```python
from build123d import *

# Parameters (mm, degrees)
SKETCH1_W           = 3
SKETCH1_H           = 400
SKETCH6_OUTSIDE_W   = 208.902
SKETCH6_OUTSIDE_H   = 208.902
CUT_EXTRUDE2_DEPTH  = 409.900966005
BOSS_EXTRUDE4_DEPTH = 7
FILLET1_R           = 10


with BuildPart() as part:
    # Sketch1 → Revolve1 (revolve)
    with BuildSketch(Plane.XY, mode=Mode.PRIVATE) as revolve1_sk:
        with Locations((58.5, 0)):
            Rectangle(SKETCH1_W, SKETCH1_H)
    revolve(revolve1_sk.sketch.rotate(Axis((0, 0, 0), (0, 1, 0)), 90), axis=Axis((0, 0, 0), (0, 1, 0)))

    # Sketch6 outside → Cut-Extrude2 (cut, through all)
    with BuildSketch(Plane(origin=(0, 200, 0), x_dir=(1, 0, 0), z_dir=(0, 1, 0))):
        Rectangle(SKETCH6_OUTSIDE_W, SKETCH6_OUTSIDE_H)
        with BuildLine():
            Line((0, -25.455844123), (53.200134751, 27.744290628))
            ThreePointArc((53.200134751, 27.744290628), (0, 60), (-53.200134751, 27.744290628))
            Line((-53.200134751, 27.744290628), (0, -25.455844123))
        make_face(mode=Mode.SUBTRACT)
    extrude(amount=-CUT_EXTRUDE2_DEPTH, mode=Mode.SUBTRACT)

    # Sketch7 → Boss-Extrude4 (add)
    with BuildSketch(Plane(origin=(0, 200, 0), x_dir=(1, 0, 0), z_dir=(0, 1, 0))):
        with BuildLine():
            Line((-35.629141961, 42.982621722), (-21.797880868, 52.667375003))
            ThreePointArc((-21.797880868, 52.667375003), (-31.660719889, 47.398299717), (-40.305086528, 40.305086528))
            Line((-40.305086528, 40.305086528), (-34.793335026, 34.793335026))
            ThreePointArc((-34.793335026, 34.793335026), (-28.516275136, 41.671387576), (-22.892502884, 49.093130862))
            Line((-22.892502884, 49.093130862), (-34.309916158, 41.09857202))
            ThreePointArc((-34.309916158, 41.09857202), (-35.91155391, 41.380983969), (-35.629141961, 42.982621722))
        make_face()
    boss_extrude4 = extrude(amount=-BOSS_EXTRUDE4_DEPTH)

    # Mirror1: Boss-Extrude4 across plane
    add(boss_extrude4.mirror(Plane.ZX))

    # Fillet1
    fillet1_edges = [part.edges().sort_by_distance(p)[0] for p in [
        (52.085351582, 200, -26.629507459),
        (-52.085351582, -200, -26.629507459),
        (52.085351582, -200, -26.629507459),
        (-52.085351582, 200, -26.629507459),
    ]]
    fillet(fillet1_edges, radius=FILLET1_R)


solid = part.part
```
The model under review builds one solid part; all positions refer to its coordinate system, in mm. A direction names the side the tool comes from. Coordinates: 2 decimals unless noted, no trailing zeros. Order: outer loops, then holes, each group sorted by start corner. A loop starts at its lowest first (then second) coordinate and runs counter-clockwise, first axis right, second up. Notation, with made-up numbers: (2.5, 21) -> (54.5, 21) arc R8 ccw to (54.5, 32) -> close; hole circle Ø9 at (77.25, -18.75). An arc over 180 degrees is marked (long way). Answer in a Markdown table with one row per item. Add a question column.
Item 1: To check wall thickness, follow probe 1 along X at (y, z) = (33, -37); probe 2 along X at (y, z) = (7, -45.5); probe 3 along Z at (x, y) = (44, -108). State the ranges of each line that lie inside material, in increasing order.
Item 2: Mouldability with a two-part tool opening along X and no side actions: class faces 1 (the cylindrical face through (-50.72, 197.15, -29.52)), 2 (the cylindrical face through (50.72, -197.15, -29.52)), 3 (the flat face through (-32, 193, -42)) as +X half, -X half, draft (parallel to the pull), parting line (faces both ways), or undercut.
Item 3: We need section A-A on y = -24.5. Write out the cut boundary in (x, z).
Item 4: We need section B-B on x = 15. Write out the cut boundary in (y, z), plus the area to 3 significant figures.
Item 5: Clearance check with flat-ended pins moving along their axes: pin 1 (1.5 mm diameter, centred on x = 31.5, z = -46.5, fed in from +Y); pin 2 (10 mm diameter, centred on x = 39.5, y = 8.5, fed in from +Z); pin 3 (6 mm diameter, centred on y = 126.5, z = -44.5, fed in from -X); pin 4 (4 mm diameter, centred on x = 29, y = -74, fed in from +Z). State where each tip first meets the part, or that it passes through.
Item 6: Machinability: for faces 4 (the cylindrical face through (-28.6, 196.55, -41.57)), 5 (the cylindrical face through (0.883, 2.8, -56.993)), 6 (the flat face through (-28.521, -196.549, -45.152)), which of the approach directions +Z, -Z, +X, -X, +Y, -Y give a long, thin tool a straight path to every point of the face, cutting with its end or side? Answer none if there is none.
Final values:
| question | item | result |
|---|---|---|
| 1 | probe 1 | x = -47.23 to -43.36, 43.36 to 47.23 |
| 1 | probe 2 | x = -39.11 to -34.33, 34.33 to 39.11 |
| 1 | probe 3 | z = -40.79 to -36.24 |
| 2 | face 1 | -X half |
| 2 | face 2 | +X half |
| 2 | face 3 | undercut |
| 3 | outline | (-53.2, -27.74) arc R60 ccw to (53.2, -27.74) -> (50.97, -25.51) arc R57 cw to (-50.97, -25.51) -> close |
| 4 | outline | (-200, -58.09) -> (200, -58.09) -> (200, -54.99) -> (-200, -54.99) -> close |
| 4 | area | 1,240 mm2 |
| 5 | pin 1 | passes through |
| 5 | pin 2 | stops at z = -35.62 |
| 5 | pin 3 | stops at x = -43.33 |
| 5 | pin 4 | stops at z = -47.83 |
| 6 | face 4 | +Z, +Y, -Y |
| 6 | face 5 | +Z |
| 6 | face 6 | +Y, -Y |
